Autodesk Inventor part; units mm, degrees
ref_plane "YZ Plane" through (0, 0, 0) normal (1, 0, 0) x (0, 1, 0)
ref_plane "XZ Plane" through (0, 0, 0) normal (0, 1, 0) x (-1, 0, 0)
ref_plane "XY Plane" through (0, 0, 0) normal (0, 0, 1) x (1, 0, 0)
sketch "Sketch1" plane through (0, 0, 0) normal (0, 1, 0) x (-1, 0, 0)
  line L0 (15, 15) -> (0, 15)
  line L1 (0, 15) -> (0, 0)
  line L2 (0, 0) -> (15, 0)
  line L3 (15, 0) -> (15, 15)
  dimension "d0" = 15
  dimension "d1" = 15
extrude "Extrusion1" add sketch "Sketch1" along normal blind 13
sketch "Sketch2" plane through (0, 13, 0) normal (0, 1, 0) x (1, 0, 0)
  line L0 (-15, -15) -> (0, -15) construction
  line L1 (0, -15) -> (0, 0) construction
  line L2 (0, 0) -> (-15, 0) construction
  line L3 (-15, 0) -> (-15, -15) construction
  line L4 (-15, 0) -> (-15, -15) construction
  line L5 (-15, -7.5) -> (0, -7.5) construction
  line L6 (-15, -7.5) -> (0, -7.5)
  line L7 (0, -7.5) -> (0, 0)
  line L8 (0, 0) -> (-15, 0)
  line L9 (-15, 0) -> (-15, -7.5)
extrude "Extrusion2" cut sketch "Sketch2" against normal blind 4.1
sketch "Sketch3" plane through (0, 13, 0) normal (0, 1, 0) x (1, 0, 0)
  line L0 (0, -7.5) -> (-15, -7.5) construction
  line L1 (-15, -7.5) -> (-15, -15) construction
  line L2 (-15, -15) -> (0, -15) construction
  line L3 (0, -15) -> (0, -7.5) construction
  line L4 (-15, -15) -> (0, -15) construction
  line L5 (-7.5, -15) -> (-7.5, -7.5) construction
  line L6 (-15, -15) -> (-7.5, -15)
  line L7 (-7.5, -15) -> (-7.5, -7.5)
  line L8 (-7.5, -7.5) -> (-15, -7.5)
  line L9 (-15, -7.5) -> (-15, -15)
  point P0 (0, 0)
extrude "Extrusion3" add sketch "Sketch3" along normal blind 1
sketch "Sketch4" plane through (0, 8.9, 0) normal (0, 1, 0) x (1, 0, 0)
  line L0 (0, 0) -> (0, -7.5) construction
  line L1 (-15, 0) -> (0, 0) construction
  line L2 (-15, -7.5) -> (-15, 0) construction
  line L3 (0, -7.5) -> (-15, -7.5) construction
  line L4 (-7.5, -7.5) -> (-7.5, 0) construction
  line L5 (-7.5, -7.5) -> (0, -7.5)
  line L6 (0, -7.5) -> (0, 0)
  line L7 (0, 0) -> (-7.5, 0)
  line L8 (-7.5, 0) -> (-7.5, -7.5)
extrude "Extrusion4" add sketch "Sketch4" along normal blind 1
sketch "Sketch5" plane through (0, 14, 0) normal (0, 1, 0) x (1, 0, 0)
  line L0 (-15, -15) -> (-7.5, -15) construction
  line L1 (-7.5, -15) -> (-7.5, -7.5) construction
  line L2 (-7.5, -7.5) -> (-15, -7.5) construction
  line L3 (-15, -7.5) -> (-15, -15) construction
  point P0 (0, 0)
  point P1 (-11.25, -11.25)
  point P2 (-11.25, -11.25)
sketch "Sketch6" plane through (0, 13, 0) normal (0, 1, 0) x (1, 0, 0)
  line L0 (-7.5, -7.5) -> (-7.5, -15) construction
  line L1 (-7.5, -15) -> (0, -15) construction
  line L2 (0, -15) -> (0, -7.5) construction
  line L3 (0, -7.5) -> (-7.5, -7.5) construction
  point P0 (0, 0)
  point P1 (-3.75, -11.25)
sketch "Sketch7" plane through (0, 9.9, 0) normal (0, 1, 0) x (1, 0, 0)
  line L0 (0, -7.5) -> (0, 0) construction
  line L1 (0, 0) -> (-7.5, 0) construction
  line L2 (-7.5, 0) -> (-7.5, -7.5) construction
  line L3 (0, -7.5) -> (-7.5, -7.5) construction
  point P0 (-3.75, -3.75)
sketch "Sketch8" plane through (0, 8.9, 0) normal (0, 1, 0) x (1, 0, 0)
  line L0 (-7.5, -7.5) -> (-7.5, 0) construction
  line L1 (-15, 0) -> (-7.5, 0) construction
  line L2 (-15, -7.5) -> (-15, 0) construction
  line L3 (-7.5, -7.5) -> (-15, -7.5) construction
  point P0 (0, 0)
  point P1 (-11.25, -3.75)
hole "Hole1" at (-11.25, 14, 11.25) direction (0, -1, 0) diameter 2.8448 depth 10.414 counterbore diameter 5.5 counterbore depth 2.85
hole "Hole2" at (-3.75, 13, 11.25) direction (0, -1, 0) diameter 2.8448 depth 10.414 counterbore diameter 5.5 counterbore depth 2.85
hole "Hole3" at (-11.25, 8.9, 3.75) direction (0, -1, 0) diameter 2.8448 depth 10.414 counterbore diameter 5.5 counterbore depth 2.85
hole "Hole4" at (-3.75, 9.9, 3.75) direction (0, -1, 0) diameter 2.8448 depth 10.414 counterbore diameter 5.5 counterbore depth 2.85
properties part number "screwprint"
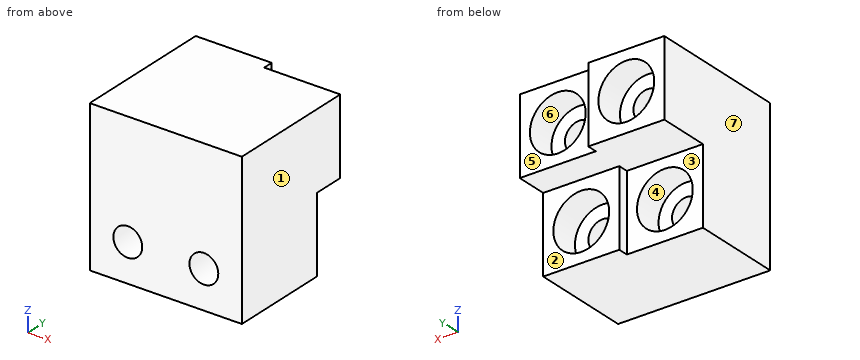
Check sheet for the modelled part. Datum: model origin and axes. Units: mm. Face numbers are marked on the shaded views. A direction names the side the tool comes from. Round coordinates to 2 decimals unless told otherwise and drop trailing zeros. Loops run counter-clockwise (first coordinate to the right, second up) from the corner with the lowest first, then second, coordinate; pieces in that order, holes last.
1. Mould release check, pull along X, two halves, no side actions. Record for the marked faces 5, 6 and 7: released by +X, released by -X, zero draft, split by the parting line, or undercut.
2. Scan lines: probe 1 along Z at (x, y) = (-3.75, 9.15); probe 2 along X at (y, z) = (7.7, 3.75); probe 3 along X at (y, z) = (3.5, 3.75). Record each from-to range of solid material in increasing order.
3. Sectioned sample at D-D on z = 11.25. Record the boundary of the cut face in (x, y), and give its area (3 significant figures).
4. Set-up check for the marked faces 1, 2, 3 and 4: record each of +Z, -Z, +X, -X, +Y, -Y from which the full face is reachable in a straight line by a thin tool's end or side.
5. Gauge pin test, flat ends, axial feed: pin 1 Ø5 at (x, z) = (-11.25, 11.25) entering from -Y; pin 2 Ø1.4 at (x, z) = (-4.5, 11) entering from +Y; pin 3 Ø2.5 at (x, z) = (-11, 11.5) entering from +Y; pin 4 Ø2 at (x, z) = (-13, 3) entering from +Y. Record the tip position at first contact, or that the pin passes through.
6. Sectioned sample at B-B on z = 3.75. Record the boundary of the cut face in (x, y).
7. Sectioned sample at A-A on x = -11.25. Record the boundary of the cut face in (y, z), and give its area (3 significant figures).
8. Sectioned sample at C-C on y = 1.5. Record the boundary of the cut face in (x, z), and give its area (3 significant figures).
Recorded:
1. face 5: zero draft
1. face 6: undercut
1. face 7: released by -X
2. probe 1: z = 0 to 1, 6.5 to 9.83, 12.67 to 15
2. probe 2: x = -15 to -14, -8.5 to -6.5, -1 to 0
2. probe 3: x = -15 to -12.67, -9.83 to -5.17, -2.33 to 0
3. outline: (-15, 0) - (0, 0) - (0, 13) - (-1, 13) - (-1, 10.15) - (-2.33, 10.15) - (-2.33, 2.59) - (-5.17, 2.59) - (-5.17, 10.15) - (-6.5, 10.15) - (-6.5, 13) - (-7.5, 13) - (-7.5, 14) - (-8.5, 14) - (-8.5, 11.15) - (-9.83, 11.15) - (-9.83, 3.59) - (-12.67, 3.59) - (-12.67, 11.15) - (-14, 11.15) - (-14, 14) - (-15, 14) - close
3. area: 128 mm2
4. face 1: +Z, -Z, +X, +Y, -Y
4. face 2: -Z, +X, -X, +Y
4. face 3: -Z, -X, +Y
4. face 4: +Y
5. pin 1: stops at y = 0
5. pin 2: stops at y = 10.15
5. pin 3: stops at y = 11.15
5. pin 4: stops at y = 8.9
6. outline: (-15, 0) - (-12.67, 0) - (-12.67, 6.05) - (-14, 6.05) - (-14, 8.9) - (-15, 8.9) - close; (-9.83, 0) - (-5.17, 0) - (-5.17, 7.05) - (-6.5, 7.05) - (-6.5, 9.9) - (-7.5, 9.9) - (-7.5, 8.9) - (-8.5, 8.9) - (-8.5, 6.05) - (-9.83, 6.05) - close; (-2.33, 0) - (0, 0) - (0, 9.9) - (-1, 9.9) - (-1, 7.05) - (-2.33, 7.05) - close
7. outline: (0, 0) - (8.9, 0) - (8.9, 1) - (6.05, 1) - (6.05, 2.33) - (0, 2.33) - close; (0, 5.17) - (6.05, 5.17) - (6.05, 6.5) - (8.9, 6.5) - (8.9, 7.5) - (14, 7.5) - (14, 8.5) - (11.15, 8.5) - (11.15, 9.83) - (3.59, 9.83) - (3.59, 12.67) - (11.15, 12.67) - (11.15, 14) - (14, 14) - (14, 15) - (0, 15) - close
7. area: 102 mm2
8. outline: (-15, 0) - (0, 0) - (0, 15) - (-15, 15) - close; hole circle Ø2.84 at (-11.25, 3.75); hole circle Ø2.84 at (-3.75, 3.75)
8. area: 212 mm2
